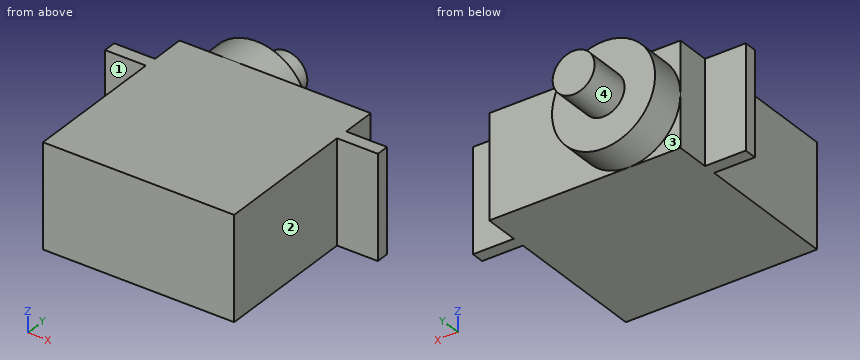
from build123d import *

# Parameters (mm, degrees)
F1_DEPTH = 12.192
F2_R     = 6.096
F3_DEPTH = 4.191
F4_R     = 2.4765
F5_DEPTH = 4.953


with BuildPart() as f1:
    # F0 (on Top) → F1 (new body)
    with BuildSketch(Plane.XY):
        Polygon((0, 17.030123), (0, 0), (22.606, 0), (22.606, 17.030123), (27.432, 17.030123), (27.432, 18.542), (22.606, 18.542), (22.606, 22.606), (0, 22.606), (0, 18.542), (-4.826, 18.542), (-4.826, 17.030123), align=None)
    extrude(amount=F1_DEPTH)

    # F2 (on face) → F3 (join)
    with BuildSketch(Plane(origin=(0, 22.606, 0), x_dir=(-1, 0, 0), z_dir=(0, 1, 0))):
        with Locations((-6.096, 6.096)):
            Circle(F2_R)
    extrude(amount=F3_DEPTH)

    # F4 (on face) → F5 (join)
    with BuildSketch(Plane(origin=(0, 26.797, 0), x_dir=(-1, 0, 0), z_dir=(0, 1, 0))):
        with Locations((-6.096, 6.096)):
            Circle(F4_R)
    extrude(amount=F5_DEPTH)


solid = f1.part
Geometry check sheet. Reference: the model listing, model coordinates, mm. Face numbers are marked on the shaded views. A direction names the side the tool comes from. Give positions to 0.01 mm unless a question says otherwise; leave off trailing zeros. Order: outer loops, then holes, each group sorted by start corner. A loop starts at its lowest first (then second) coordinate and runs counter-clockwise, first axis right, second up. Notation, with made-up numbers: M 11.5,30 L 49.5,30 A33 ccw 49.5,64 Z; hole C -26.75,51.5 d2. An arc over 180 degrees is marked long. Use a Markdown table: item, result.
Item 1: Material ranges on line 1 along X through (y, z) = (14.5, 8.75); line 2 along Y through (x, z) = (3, 8.25), recorded low to high.
Answers follow:
| item | result |
|---|---|
| line 1 | x = 0 to 22.61 |
| line 2 | y = 0 to 26.8 |
Item 2: Section check A-A (z = 7). Record the cut outline in (x, y), and give its area (3 significant figures).
Answers follow:
| item | result |
|---|---|
| outline | M -4.83,17.03 L 0,17.03 L 0,0 L 22.61,0 L 22.61,17.03 L 27.43,17.03 L 27.43,18.54 L 22.61,18.54 L 22.61,22.61 L 12.12,22.61 L 12.12,26.8 L 8.4,26.8 L 8.4,31.75 L 3.79,31.75 L 3.79,26.8 L 0.07,26.8 L 0.07,22.61 L 0,22.61 L 0,18.54 L -4.83,18.54 Z |
| area | 599 mm2 |
Item 3: Depth check by flat-ended pin: P1, Ø2.5, axis at x = 24, z = 7.5, coming from the +Y side; P2, Ø1.4, axis at x = -3, z = 6.5, coming from the -Y side; P3, Ø4.5, axis at y = 21, z = 8.5, coming from the -X side. Enter the tip coordinate at first touch or a pass-through.
Answers follow:
| item | result |
|---|---|
| P1 | stops at y = 18.54 |
| P2 | stops at y = 17.03 |
| P3 | stops at x = 0 |
Item 4: Tool access check on the marked faces 1, 2, 3 and 4. Record the directions out of +Z, -Z, +X, -X, +Y, -Y that give a thin tool (end or side, any length) a straight path to the whole face; none if there is none.
Answers follow:
| item | result |
|---|---|
| face 1 | +Z, -Z, -X, -Y |
| face 2 | +Z, -Z, +X, -Y |
| face 3 | -Z, -X, +Y |
| face 4 | +Y |
Item 5: Section check B-B (x = 1). Record the cut outline in (y, z).
Answers follow:
| item | result |
|---|---|
| outline | M 0,0 L 22.61,0 L 22.61,2.75 L 26.8,2.75 L 26.8,9.44 L 22.61,9.44 L 22.61,12.19 L 0,12.19 Z |
Item 6: Section check C-C (y = 23.5). Record the cut outline in (x, z), and give its area (3 significant figures).
Answers follow:
| item | result |
|---|---|
| outline | C 6.1,6.1 d12.19 |
| area | 117 mm2 |
Item 7: Section check D-D (z = 9.5). Record the cut outline in (x, y).
Answers follow:
| item | result |
|---|---|
| outline | M -4.83,17.03 L 0,17.03 L 0,0 L 22.61,0 L 22.61,17.03 L 27.43,17.03 L 27.43,18.54 L 22.61,18.54 L 22.61,22.61 L 11.15,22.61 L 11.15,26.8 L 1.04,26.8 L 1.04,22.61 L 0,22.61 L 0,18.54 L -4.83,18.54 Z |
